from build123d import *

# Parameters (mm, degrees)
F0_W     = 250
F0_H     = 10
F1_DEPTH = 60
F2_START = 5
F0_H_2   = 40
F2_DEPTH = 50
F3_R     = 10
F4_DEPTH = 60.001


with BuildPart() as f1:
    # F0 (on Right) → F1 (new body)
    with BuildSketch(Plane.YZ):
        with Locations((0, 25)):
            Rectangle(F0_W, F0_H)
        with BuildLine():
            Line((-125, 20), (-125, 30))
            ThreePointArc((-125, 30), (-155, 0), (-125, -30))
            Line((-125, -30), (-125, -20))
            ThreePointArc((-125, -20), (-145, 0), (-125, 20))
        make_face()
        with BuildLine():
            ThreePointArc((125, -30), (155, 0), (125, 30))
            Line((125, 30), (125, 20))
            ThreePointArc((125, 20), (145, 0), (125, -20))
            Line((125, -20), (125, -30))
        make_face()
        with Locations((0, -25)):
            Rectangle(F0_W, F0_H)
    extrude(amount=F1_DEPTH)

    # F0 (on Right) → F2 (join)
    with BuildSketch(Plane.YZ.offset(F2_START)):
        Rectangle(F0_W, F0_H_2)
        with BuildLine():
            ThreePointArc((125, -20), (145, 0), (125, 20))
            Line((125, 20), (125, -20))
        make_face()
        with BuildLine():
            Line((-125, -20), (-125, 20))
            ThreePointArc((-125, 20), (-145, 0), (-125, -20))
        make_face()
    extrude(amount=F2_DEPTH)

    # F3 (on Right) → F4 (cut, through all)
    with BuildSketch(Plane.YZ):
        with Locations((-125, 0)):
            Circle(F3_R)
        with Locations((125, 0)):
            Circle(F3_R)
    extrude(amount=F4_DEPTH, mode=Mode.SUBTRACT)


solid = f1.part
Can you work these out from the model? Positions are in its coordinate system, mm. A direction names the side the tool comes from. Give positions to 0.01 mm unless a question says otherwise; leave off trailing zeros. Loops run counter-clockwise (first coordinate to the right, second up) from the corner with the lowest first, then second, coordinate; pieces in that order, holes last. Notation, with made-up numbers: (-13.75, 33) - (25.25, 33) arc R27 ccw to (25.25, 71) - close; hole circle Ø4 at (67, 79). An arc over 180 degrees is marked (long way). Return JSON: item names as keys, results as strings.
1. I'm going to push flat-ended pins straight in: pin 1 Ø3 at (y, z) = (-6, -3) entering from +X; pin 2 Ø1 at (x, z) = (43, -9) entering from -Y; pin 3 Ø10 at (x, z) = (16.5, 3.5) entering from +Y. Where does each tip first touch, or does it pass through?
Output values:
{"pin 1": "stops at x = 55", "pin 2": "stops at y = -153.77", "pin 3": "stops at y = 155"}
2. I want a section at C-C on y = 46. Please give me the cut outline in (x, z), and give its area (3 significant figures).
Output values:
{"outline": "(0, -30) - (60, -30) - (60, -20) - (55, -20) - (55, 20) - (60, 20) - (60, 30) - (0, 30) - (0, 20) - (5, 20) - (5, -20) - (0, -20) - close", "area": "3,200 mm²"}
3. We'd pull the mould along Z, two halves only. Please class faces 1 (the face through (30, 115, 0)), 2 (the face through (29.58, -154.993, 0.66)), 3 (the face through (2, 145, 0)), 4 (the face through (30, -2, 30)): +Z half, -Z half, draft (parallel to the pull), parting line (faces both ways), or undercut.
Output values:
{"face 1": "undercut", "face 2": "parting line", "face 3": "undercut", "face 4": "+Z half"}
4. For faces 5 (the face through (55, -2, 0)), 6 (the face through (2, -2, 20)), 7 (the face through (29.58, 154.993, -0.66)), which set-ups out of +Z, -Z, +X, -X, +Y, -Y let a thin tool reach every point of the face, with its end or its side?
Output values:
{"face 5": "+X", "face 6": "-X", "face 7": "+X, -X, +Y"}
5. If I drill on line 1 (Y direction, x = 36, z = 0); line 2 (Z direction, x = 4, y = 25.5); line 3 (Z direction, x = 15.5, y = -125), over which ranges is the centre line in solid material (lowest first)?
Output values:
{"line 1": "y = -155 to -135, -115 to 115, 135 to 155", "line 2": "z = -30 to -20, 20 to 30", "line 3": "z = -30 to -10, 10 to 30"}
6. I want a section at B-B on x = 47. Please give me the cut outline in (y, z).
Output values:
{"outline": "(-125, -30) - (125, -30) arc R30 ccw to (125, 30) - (-125, 30) arc R30 ccw to start; hole circle Ø20 at (-125, 0); hole circle Ø20 at (125, 0)"}
7. I want a section at A-A on z = 0. Please give me the cut outline in (x, y), and give its area (3 significant figures).
Output values:
{"outline": "(0, -155) - (60, -155) - (60, -145) - (55, -145) - (55, -135) - (5, -135) - (5, -145) - (0, -145) - close; (0, 145) - (5, 145) - (5, 135) - (55, 135) - (55, 145) - (60, 145) - (60, 155) - (0, 155) - close; (5, -115) - (55, -115) - (55, 115) - (5, 115) - close", "area": "13,700 mm²"}
